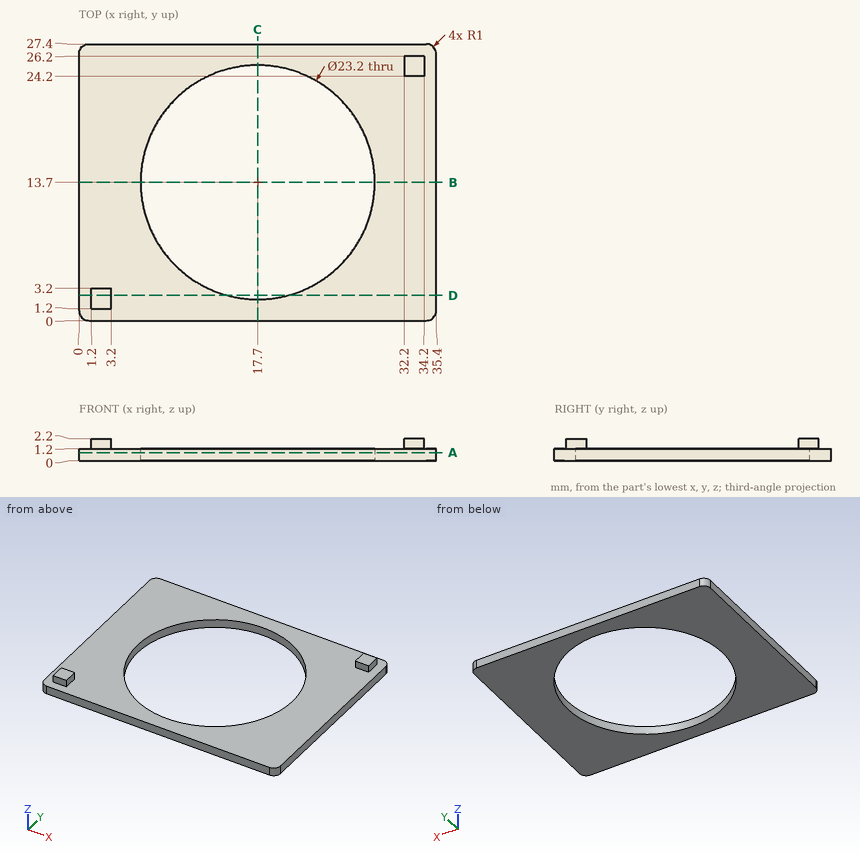
The figure shows three views and two pictorial views of one solid part (mm, origin at its lowest corner). Answer the questions. Give positions to 0.01 mm unless a question says otherwise; leave off trailing zeros. Loops run counter-clockwise (first coordinate to the right, second up) from the corner with the lowest first, then second, coordinate; pieces in that order, holes last. Notation, with made-up numbers: (18, -24.75) -> (22, -24.75) arc R24 cw to (22, -9.75) -> close; hole circle Ø3 at (-34.5, 77.5). An arc over 180 degrees is marked (long way). Use CSV: the item, a comma, the result in double quotes.
1. The part is cut by section D-D (y = 2.5). Write down the section's boundary in (x, z), then the cut area to 3 significant figures.
Found:
outline,"(0, 0) -> (14.68, 0) -> (14.68, 1.2) -> (3.2, 1.2) -> (3.2, 2.2) -> (1.2, 2.2) -> (1.2, 1.2) -> (0, 1.2) -> close; (20.72, 0) -> (35.4, 0) -> (35.4, 1.2) -> (20.72, 1.2) -> close"
area,"37.2 mm^2"
2. The part is cut by section A-A (z = 0.8). Write down the section's boundary in (x, y), then the cut area to 3 significant figures.
Found:
outline,"(0, 1) arc R1 ccw to (1, 0) -> (34.4, 0) arc R1 ccw to (35.4, 1) -> (35.4, 26.4) arc R1 ccw to (34.4, 27.4) -> (1, 27.4) arc R1 ccw to (0, 26.4) -> close; hole circle Ø23.2 at (17.7, 13.7)"
area,"546 mm^2"
3. Straight lines are drawn through the part: line 1 (Y direction, x = 17.7, z = 0.8); line 2 (X direction, y = 19.75, z = 0.6); line 3 (Z direction, x = 2.5, y = 9.75). For each, find the intervals that lie inside material, in ascending order.
Found:
line 1,"0 to 2.1, 25.3 to 27.4"
line 2,"0 to 7.8, 27.6 to 35.4"
line 3,"0 to 1.2"
4. The part is cut by section C-C (x = 17.7). Write down the section's boundary in (y, z).
Found:
outline,"(0, 0) -> (2.1, 0) -> (2.1, 1.2) -> (0, 1.2) -> close; (25.3, 0) -> (27.4, 0) -> (27.4, 1.2) -> (25.3, 1.2) -> close"
5. Flat-ended cylindrical pins translate along their axes: pin 1 Ø0.8 at (y, z) = (25.5, 1.5) entering from -X; pin 2 Ø0.5 at (y, z) = (2.5, 1.5) entering from +X; pin 3 Ø0.8 at (x, z) = (33, 2) entering from -Y; pin 4 Ø1 at (y, z) = (12, 2) entering from +X. Find the tip coordinate at first contact, or state that the pin passes through.
Found:
pin 1,"x = 0"
pin 2,"x = 3.2"
pin 3,"y = 24.2"
pin 4,"through"
6. The part is cut by section B-B (y = 13.7). Write down the section's boundary in (x, z).
Found:
outline,"(0, 0) -> (6.1, 0) -> (6.1, 1.2) -> (0, 1.2) -> close; (29.3, 0) -> (35.4, 0) -> (35.4, 1.2) -> (29.3, 1.2) -> close"
